Here's how the part is built. I have some questions about the finished solid (model axes, mm). Round coordinates to 2 decimals unless told otherwise and drop trailing zeros. Order: outer loops, then holes, each group sorted by start corner. A loop starts at its lowest first (then second) coordinate and runs counter-clockwise, first axis right, second up. Notation, with made-up numbers: (-23, 24) - (35, 24) arc R23 cw to (35, 38) - close; hole circle Ø9 at (73.5, 68.5). An arc over 180 degrees is marked (long way). Answer as a JSON object with one key per item and string values.
```python
from build123d import *

# Parameters (mm, degrees)
FLANGE_START                 = 98
SKETCH1_W                    = 94
SKETCH1_H                    = 134
FLANGE_DEPTH                 = 3
PORT_AND_M3_HOLES_DEPTH      = 236.072329295
PORT_AND_M3_HOLES_DEPTH_BACK = 236.072329295
SKETCH2_R                    = 1.7
SKETCH2_W                    = 60
SKETCH2_H                    = 100


with BuildPart() as part:
    # Sketch1 → flange (new body)
    with BuildSketch(Plane(origin=(0, 0, 0), x_dir=(0, 0, -1), z_dir=(1, 0, 0)).offset(FLANGE_START)):
        with Locations((0, 140)):
            Rectangle(SKETCH1_W, SKETCH1_H)
    extrude(amount=FLANGE_DEPTH)

    # Sketch2 → Port_and_M3_holes (cut, two sides: drawn at the far end of the back side and taken through both)
    with BuildSketch(Plane(origin=(0, 0, 0), x_dir=(0, 0, -1), z_dir=(1, 0, 0)).offset(-PORT_AND_M3_HOLES_DEPTH_BACK)):
        with Locations((40, 80)):
            Circle(SKETCH2_R)
        with Locations((-40, 80)):
            Circle(SKETCH2_R)
        with Locations((40, 200)):
            Circle(SKETCH2_R)
        with Locations((-40, 200)):
            Circle(SKETCH2_R)
        with Locations((0, 140)):
            Rectangle(SKETCH2_W, SKETCH2_H)
    extrude(amount=PORT_AND_M3_HOLES_DEPTH + PORT_AND_M3_HOLES_DEPTH_BACK, mode=Mode.SUBTRACT)


solid = part.part
```
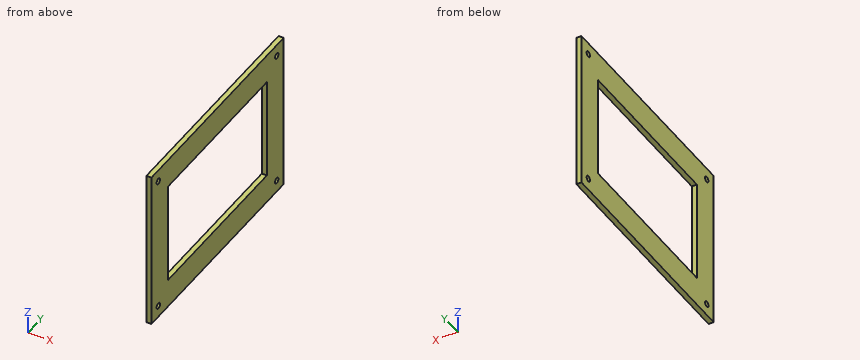
1. If I drill on L1, parallel to Y at x = 98.6, z = -40; L2, parallel to Z at x = 100.3, y = 80; L3, parallel to Z at x = 100.5, y = 97, over which ranges is the centre line in solid material (lowest first)? Write a range as [from, to].
Responses:
{"L1": "[73, 78.3], [81.7, 198.3], [201.7, 207]", "L2": "[-47, -41.7], [-38.3, 38.3], [41.7, 47]", "L3": "[-47, -30], [30, 47]"}
2. Imagine slicing it at D-D (x = 98.5). List the corners of the cut face in (y, z) for me.
Responses:
{"outline": "(73, -47) - (207, -47) - (207, 47) - (73, 47) - close; hole circle Ø3.4 at (80, -40); hole circle Ø3.4 at (80, 40); hole (90, -30) - (190, -30) - (190, 30) - (90, 30) - close; hole circle Ø3.4 at (200, -40); hole circle Ø3.4 at (200, 40)"}
3. Imagine slicing it at B-B (z = -40). List the corners of the cut face in (x, y) for me.
Responses:
{"outline": "(98, 73) - (101, 73) - (101, 78.3) - (98, 78.3) - close; (98, 81.7) - (101, 81.7) - (101, 198.3) - (98, 198.3) - close; (98, 201.7) - (101, 201.7) - (101, 207) - (98, 207) - close"}
4. Imagine slicing it at C-C (y = 121.5). List the corners of the cut face in (x, z) for me, plus the area to 3 significant figures.
Responses:
{"outline": "(98, -47) - (101, -47) - (101, -30) - (98, -30) - close; (98, 30) - (101, 30) - (101, 47) - (98, 47) - close", "area": "102 mm2"}
5. Imagine slicing it at A-A (y = 200). List the corners of the cut face in (x, z) for me.
Responses:
{"outline": "(98, -47) - (101, -47) - (101, -41.7) - (98, -41.7) - close; (98, -38.3) - (101, -38.3) - (101, 38.3) - (98, 38.3) - close; (98, 41.7) - (101, 41.7) - (101, 47) - (98, 47) - close"}
